```python
from build123d import *

# Parameters (mm, degrees)
SKETCH_1_W      = 41.9
SKETCH_1_H      = 47.1
SKETCH_1_R      = 1.5875
EXTRUDE_1_DEPTH = 1.6
SKETCH_2_W      = 3.15
SKETCH_2_H      = 4
SKETCH_2_W_2    = 4
SKETCH_2_H_2    = 3.15
EXTRUDE_2_DEPTH = 2
SKETCH_3_W      = 8.83
SKETCH_3_H      = 3.21
EXTRUDE_3_DEPTH = 5
SKETCH_4_W      = 4.77
SKETCH_4_H      = 19.56
EXTRUDE_4_DEPTH = 5
SKETCH_5_W      = 14
SKETCH_5_H      = 14
SKETCH_5_W_2    = 13.1
SKETCH_5_H_2    = 8.1
SKETCH_5_W_3    = 8
SKETCH_5_H_3    = 6
EXTRUDE_5_DEPTH = 1


with BuildPart() as part:
    # 草图1 → 凸台-拉伸1 (new body)
    with BuildSketch(Plane(origin=(0, 0, 0), x_dir=(1, 0, 0), z_dir=(0, 1, 0))):
        with Locations((20.95, 23.55)):
            Rectangle(SKETCH_1_W, SKETCH_1_H)
        with Locations(Location((4.34, 42.61, 0), (0, 0, 270))):
            Circle(SKETCH_1_R, mode=Mode.SUBTRACT)
        with Locations(Location((37.59, 42.61, 0), (0, 0, 270))):
            Circle(SKETCH_1_R, mode=Mode.SUBTRACT)
        with Locations(Location((37.59, 4.47, 0), (0, 0, 270))):
            Circle(SKETCH_1_R, mode=Mode.SUBTRACT)
        with Locations(Location((4.34, 4.47, 0), (0, 0, 270))):
            Circle(SKETCH_1_R, mode=Mode.SUBTRACT)
    extrude(amount=EXTRUDE_1_DEPTH)

    # 草图2 → 凸台-拉伸2 (add)
    with BuildSketch(Plane(origin=(0, 1.6, 0), x_dir=(1, 0, 0), z_dir=(0, 1, 0))):
        with Locations((8.325, 37.28)):
            Rectangle(SKETCH_2_W, SKETCH_2_H)
        with Locations((10.23, 44.665)):
            Rectangle(SKETCH_2_W_2, SKETCH_2_H_2)
    extrude(amount=EXTRUDE_2_DEPTH)

    # 草图3 → 凸台-拉伸3 (add)
    with BuildSketch(Plane(origin=(0, 1.6, 0), x_dir=(1, 0, 0), z_dir=(0, 1, 0))):
        with Locations((36.645, 10.795)):
            Rectangle(SKETCH_3_W, SKETCH_3_H)
    extrude(amount=EXTRUDE_3_DEPTH)

    # 草图4 → 凸台-拉伸4 (add)
    with BuildSketch(Plane.XZ):
        with Locations((4.155, -23.5)):
            Rectangle(SKETCH_4_W, SKETCH_4_H)
        with Locations((37.745, -23.5)):
            Rectangle(SKETCH_4_W, SKETCH_4_H)
    extrude(amount=EXTRUDE_4_DEPTH)

    # 草图5 → 凸台-拉伸5 (add)
    with BuildSketch(Plane(origin=(0, 1.6, 0), x_dir=(1, 0, 0), z_dir=(0, 1, 0))):
        with Locations((21, 27.2)):
            Rectangle(SKETCH_5_W, SKETCH_5_H)
        with Locations((19.35, 9.35)):
            Rectangle(SKETCH_5_W_2, SKETCH_5_H_2)
        with Locations((14.4, 37.7)):
            Rectangle(SKETCH_5_W_3, SKETCH_5_H_3)
    extrude(amount=EXTRUDE_5_DEPTH)


solid = part.part
```
Check sheet for the modelled part. Datum: model origin and axes. Units: mm. A direction names the side the tool comes from. Round coordinates to 2 decimals unless told otherwise and drop trailing zeros. Loops run counter-clockwise (first coordinate to the right, second up) from the corner with the lowest first, then second, coordinate; pieces in that order, holes last. Notation, with made-up numbers: (77.5, -28) - (121.5, -28) arc R21 cw to (121.5, -16) - close; hole circle Ø4 at (61, 8.5). An arc over 180 degrees is marked (long way). Write item = value, one per line. Start each with the question number.
Q1. Section check D-D (x = 11). Record the boundary of the cut face in (y, z).
Q2. Release check for a two-part mould opening along X. For faces 5 (the face through (37.66, 0.789, -44.196)), 6 (the face through (8.23, 3, -45)), 7 (the face through (10, 3.6, -45)), 8 (the face through (41.06, 4, -11)) record: pulls with the +X half, pulls with the -X half, needs draft (parallel to the pull), parting line crosses it, or undercut.
Q3. Depth check by flat-ended pin: P1, Ø2, axis at y = 3, z = -44.5, coming from the -X side; P2, Ø0.6, axis at x = 10.5, y = 3, coming from the +Z side; P3, Ø4, axis at x = 17.5, z = -15.5, coming from the -Y side. Enter the tip coordinate at first touch or a pass-through.
Q4. Section check B-B (y = -3.25). Record the boundary of the cut face in (x, z), plus the area to 3 significant figures.
Q5. Access from +Z, -Z, +X, -X, +Y, -Y to the whole of each face (thin tool, end or side, straight path). Record for faces 1 (the face through (12.23, 3, -45)), 2 (the face through (6.54, -2, -24)), 3 (the face through (1.77, -2, -24)), 4 (the face through (14, 2, -40.7)).
Q6. Thickness scan on L1, parallel to X at y = 0.6, z = -4.47; L2, parallel to X at y = -4.5, z = -29; L3, parallel to Y at x = 34, z = -21.5. Record the ranges inside material, lowest first.
Q7. Section check A-A (x = 4.34). Record the boundary of the cut face in (y, z).
Q8. Section check C-C (z = -16.5). Record the boundary of the cut face in (x, y).
Derived:
q1.outline = (0, -47.1) - (1.6, -47.1) - (1.6, -46.24) - (3.6, -46.24) - (3.6, -43.09) - (1.6, -43.09) - (1.6, -40.7) - (2.6, -40.7) - (2.6, -34.7) - (1.6, -34.7) - (1.6, 0) - (0, 0) - close
q2.face_5 = undercut
q2.face_6 = pulls with the -X half
q2.face_7 = needs draft
q2.face_8 = pulls with the +X half
q3.P1 = 8.23
q3.P2 = -43.09
q3.P3 = 0
q4.outline = (1.77, -33.28) - (6.54, -33.28) - (6.54, -13.72) - (1.77, -13.72) - close; (35.36, -33.28) - (40.13, -33.28) - (40.13, -13.72) - (35.36, -13.72) - close
q4.area = 187 mm^2
q5.face_1 = -Z, +X, +Y
q5.face_2 = +Z, -Z, -Y
q5.face_3 = +Z, -Z, -X, -Y
q5.face_4 = +X, -X, +Y
q6.L1 = 0 to 2.75, 5.93 to 36, 39.18 to 41.9
q6.L2 = 1.77 to 6.54, 35.36 to 40.13
q6.L3 = 0 to 1.6
q7.outline = (-5, -33.28) - (0, -33.28) - (0, -41.02) - (1.6, -41.02) - (1.6, -6.06) - (0, -6.06) - (0, -13.72) - (-5, -13.72) - close; (0, -47.1) - (1.6, -47.1) - (1.6, -44.2) - (0, -44.2) - close; (0, -2.88) - (1.6, -2.88) - (1.6, 0) - (0, 0) - close
q8.outline = (0, 0) - (1.77, 0) - (1.77, -5) - (6.54, -5) - (6.54, 0) - (35.36, 0) - (35.36, -5) - (40.13, -5) - (40.13, 0) - (41.9, 0) - (41.9, 1.6) - (0, 1.6) - close
